Can you work these out from the drawing? Everything is in mm from the part's minimum corner. A direction names the side the tool comes from. Coordinates: 2 decimals unless noted, no trailing zeros. Order: outer loops, then holes, each group sorted by start corner. A loop starts at its lowest first (then second) coordinate and runs counter-clockwise, first axis right, second up. Notation, with made-up numbers: (30, 2.25) -> (66, 2.25) arc R21 ccw to (66, 16.25) -> close; hole circle Ø9 at (45, 43). An arc over 180 degrees is marked (long way). Put each result on its own line as item: value. Start each with the question number.
Q1. If we section it at A-A (z = 3): Please give me the cut outline in (x, y).
Q2. Will these pins go through, and if not, where does the flat tip stop? pin 1 (2 mm diameter, centred on x = 13, y = 8.5, fed in from +Z); pin 2 (1.5 mm diameter, centred on x = 8.5, y = 10.5, fed in from +Z); pin 3 (4 mm diameter, centred on y = 10, z = 14.5, fed in from -X); pin 4 (1 mm diameter, centred on x = 5.5, y = 5.5, fed in from -Z).
Q3. Please list where these lines run through material, in increasing order: line 1 along Y through (x, z) = (20, 24.5); line 2 along X through (y, z) = (6, 13); line 3 along X through (y, z) = (6.2, 27).
Q4. We'd pull the mould along Z, two halves only. Please class the marked faces 3, 4 and 5: +Z half, -Z half, draft (parallel to the pull), parting line (faces both ways), or undercut.
Q5. For the marked faces 1 and 2, which set-ups out of +Z, -Z, +X, -X, +Y, -Y let a thin tool reach every point of the face, with its end or its side?
Q6. If we section it at C-C (y = 6.5): Please give me the cut outline in (x, z).
Q7. If we section it at D-D (x = 15): Please give me the cut outline in (y, z), and give its area (4 significant figures).
Q8. If we section it at B-B (x = 27): Please give me the cut outline in (y, z), and give its area (3 significant figures).
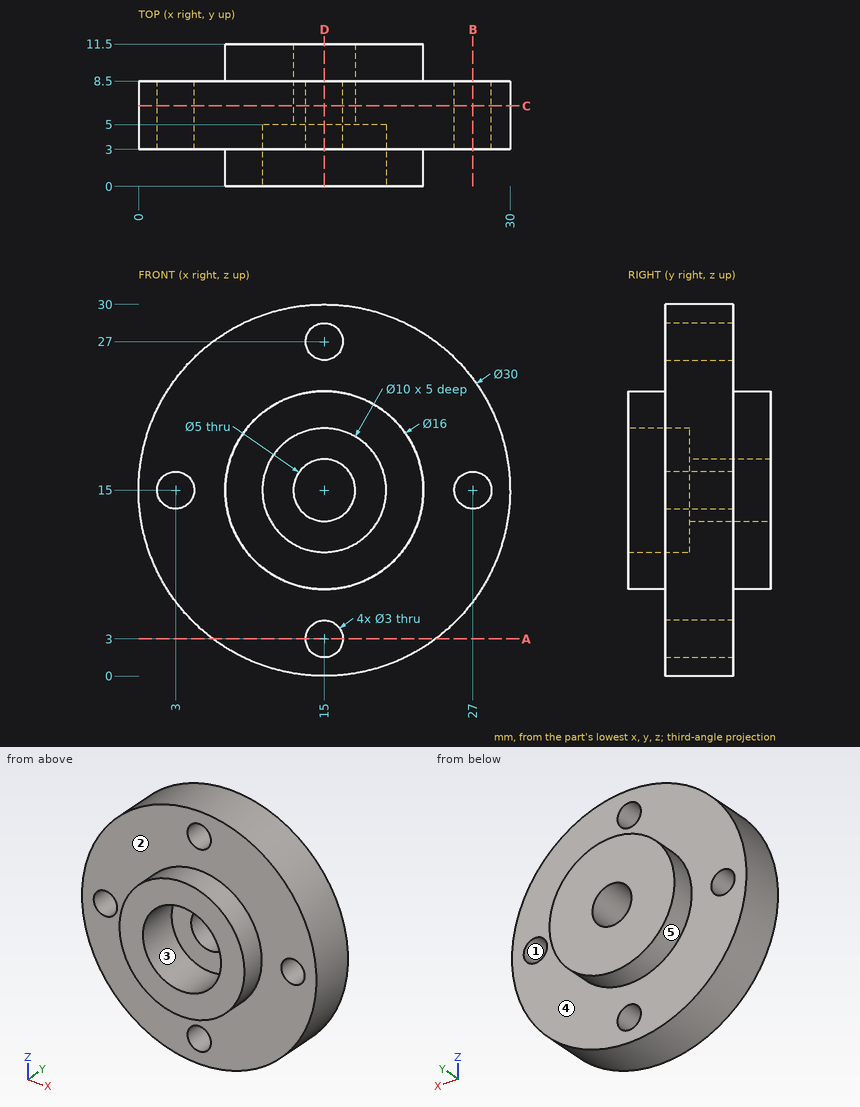
The answers:
1. outline: (6, 3) -> (13.5, 3) -> (13.5, 8.5) -> (6, 8.5) -> close; (16.5, 3) -> (24, 3) -> (24, 8.5) -> (16.5, 8.5) -> close
2. pin 1: z = 29.97
2. pin 2: z = 20.56
2. pin 3: x = 0
2. pin 4: z = 3
3. line 1: 3 to 8.5
3. line 2: 0.13 to 13.5, 16.5 to 29.87
3. line 3: 6 to 13.5, 16.5 to 24
4. face 3: undercut
4. face 4: draft
4. face 5: parting line
5. face 1: +Y, -Y
5. face 2: -Y
6. outline: circle Ø30 at (15, 15); hole circle Ø3 at (3, 15); hole circle Ø5 at (15, 15); hole circle Ø3 at (15, 3); hole circle Ø3 at (15, 27); hole circle Ø3 at (27, 15)
7. outline: (0, 7) -> (3, 7) -> (3, 4.5) -> (8.5, 4.5) -> (8.5, 7) -> (11.5, 7) -> (11.5, 12.5) -> (5, 12.5) -> (5, 10) -> (0, 10) -> close; (0, 20) -> (5, 20) -> (5, 17.5) -> (11.5, 17.5) -> (11.5, 23) -> (8.5, 23) -> (8.5, 25.5) -> (3, 25.5) -> (3, 23) -> (0, 23) -> close; (3, 0) -> (8.5, 0) -> (8.5, 1.5) -> (3, 1.5) -> close; (3, 28.5) -> (8.5, 28.5) -> (8.5, 30) -> (3, 30) -> close
7. area: 145.5 mm^2
8. outline: (3, 6) -> (8.5, 6) -> (8.5, 13.5) -> (3, 13.5) -> close; (3, 16.5) -> (8.5, 16.5) -> (8.5, 24) -> (3, 24) -> close
8. area: 82.5 mm^2
